Drawing for the job (mm, zero at the part's lowest x, y, z). Give positions to 0.01 mm unless a question says otherwise; leave off trailing zeros. Write each loop counter-clockwise with the first axis right and the second up, starting at its lowest first coordinate (ties: lowest second). Pieces come first, ordered by that corner, then holes.
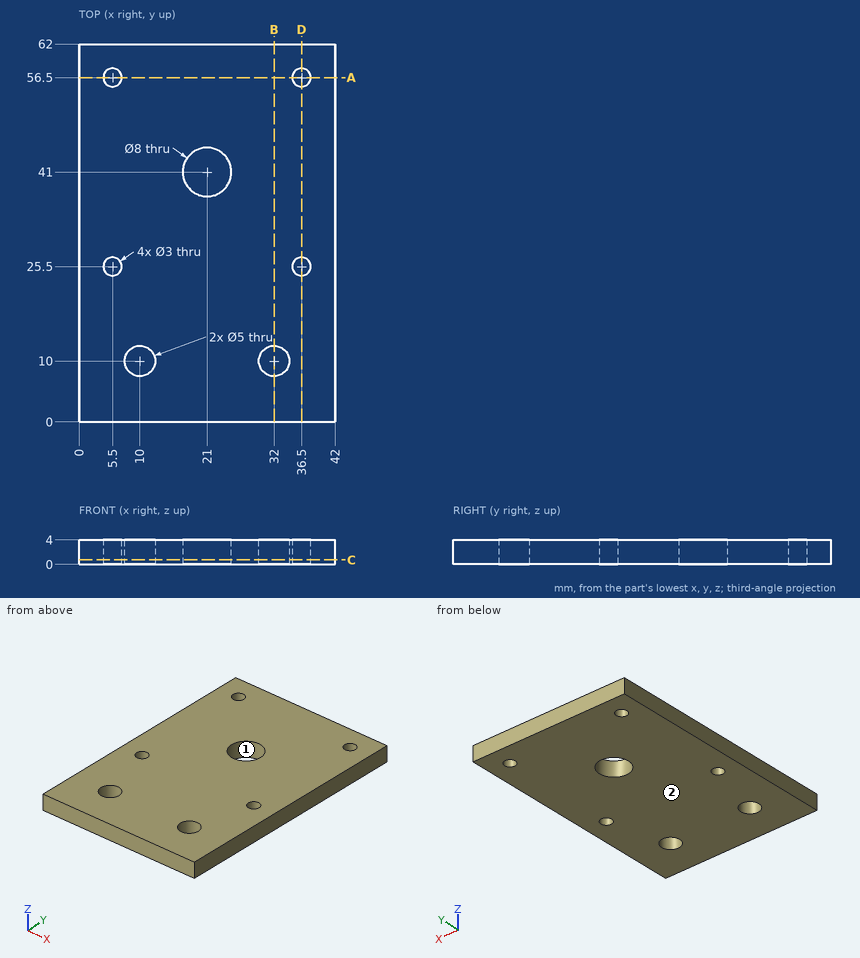
1. Slice it at B-B, the plane x = 32. Write the cut outline in (y, z).
Calculated:
outline: (0, 0) - (7.5, 0) - (7.5, 4) - (0, 4) - close; (12.5, 0) - (62, 0) - (62, 4) - (12.5, 4) - close
2. Slice it at D-D, the plane x = 36.5. Write the cut outline in (y, z), and give its area (3 significant figures).
Calculated:
outline: (0, 0) - (24, 0) - (24, 4) - (0, 4) - close; (27, 0) - (55, 0) - (55, 4) - (27, 4) - close; (58, 0) - (62, 0) - (62, 4) - (58, 4) - close
area: 224 mm2
3. Pull direction Y, two halves, no side cores. Call the marked faces 1 and 2: +Y half, -Y half, draft (parallel to the pull), parting line (faces both ways), or undercut.
Calculated:
face 1: undercut
face 2: draft
4. Slice it at C-C, the plane z = 0.75. Write the cut outline in (x, y).
Calculated:
outline: (0, 0) - (42, 0) - (42, 62) - (0, 62) - close; hole circle Ø3 at (5.5, 25.5); hole circle Ø3 at (5.5, 56.5); hole circle Ø5 at (10, 10); hole circle Ø8 at (21, 41); hole circle Ø5 at (32, 10); hole circle Ø3 at (36.5, 25.5); hole circle Ø3 at (36.5, 56.5)
5. Slice it at A-A, the plane y = 56.5. Write the cut outline in (x, z), and give its area (3 significant figures).
Calculated:
outline: (0, 0) - (4, 0) - (4, 4) - (0, 4) - close; (7, 0) - (35, 0) - (35, 4) - (7, 4) - close; (38, 0) - (42, 0) - (42, 4) - (38, 4) - close
area: 144 mm2
6. Probe probe 1 along Y at (x, z) = (5.5, 2.1); probe 2 along Y at (x, z) = (10, 2.45); probe 3 along Y at (x, z) = (21, 1.35). List the from-to ranges inside material, lowest first.
Calculated:
probe 1: y = 0 to 24, 27 to 55, 58 to 62
probe 2: y = 0 to 7.5, 12.5 to 62
probe 3: y = 0 to 37, 45 to 62
